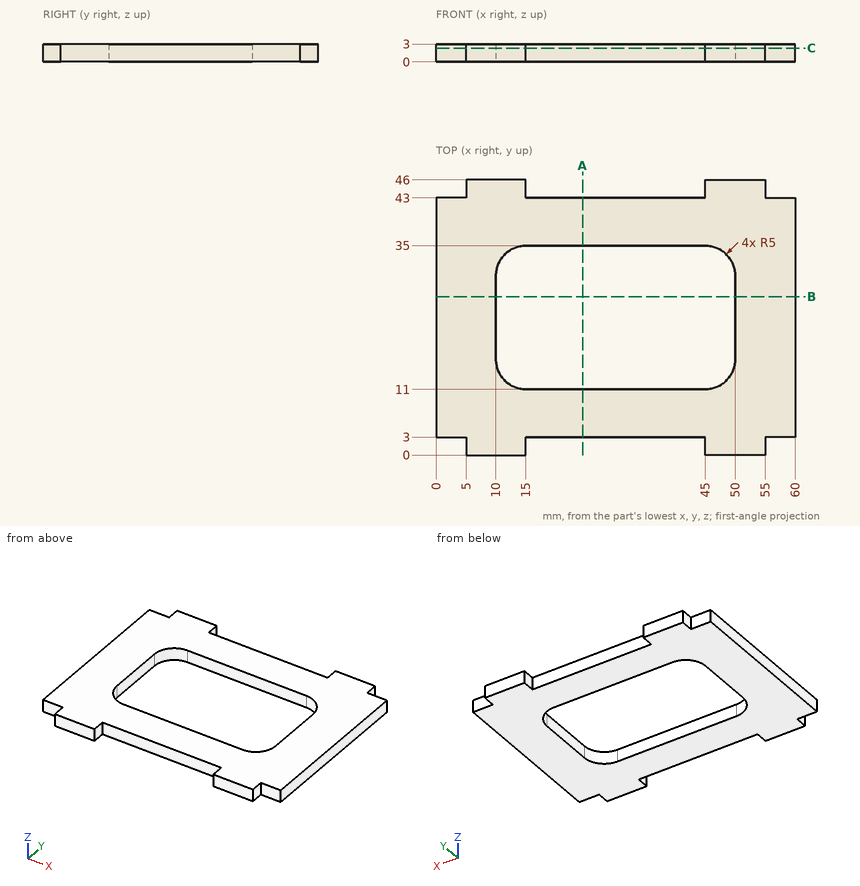
Print and shaded views of the part. All mm, measured from the part's lowest x, y and z. Coordinates: 2 decimals unless noted, no trailing zeros. Order: outer loops, then holes, each group sorted by start corner. A loop starts at its lowest first (then second) coordinate and runs counter-clockwise, first axis right, second up. Notation, with made-up numbers: (46.5, -21) - (64.5, -21) arc R14 cw to (64.5, -10) - close; hole circle Ø2 at (-6, 71.5). An arc over 180 degrees is marked (long way). Return JSON: item names as keys, results as strings. Group by question number.
Item 1: Cut at C-C (z = 2.3). List the corners of the cut face in (x, y).
Item 2: Drill centre lines: probe 1 along X at (y, z) = (23.5, 0.5); probe 2 along Y at (x, z) = (17.5, 0.85); probe 3 along X at (y, z) = (44, 0.9). Where is each one in solid material? Low to high. Write a range as from..to.
Item 3: Cut at B-B (y = 26.5). List the corners of the cut face in (x, z), plus the area to 3 significant figures.
Item 4: Pin check, flat tips, straight feed: pin 1 (1.5 mm diameter, centred on y = 1.5, z = 2, fed in from +X); pin 2 (1.5 mm diameter, centred on x = 37.5, z = 1.5, fed in from -Y). Stop position of each tip, or through.
Item 5: Cut at A-A (x = 24.5). List the corners of the cut face in (y, z).
Check values:
{
 "1": {"outline": "(0, 3) - (5, 3) - (5, 0) - (15, 0) - (15, 3) - (45, 3) - (45, 0) - (55, 0) - (55, 3) - (60, 3) - (60, 43) - (55, 43) - (55, 46) - (45, 46) - (45, 43) - (15, 43) - (15, 46) - (5, 46) - (5, 43) - (0, 43) - close; hole (10, 16) arc R5 ccw to (15, 11) - (45, 11) arc R5 ccw to (50, 16) - (50, 30) arc R5 ccw to (45, 35) - (15, 35) arc R5 ccw to (10, 30) - close"},
 "2": {"probe 1": "x = 0..10, 50..60", "probe 2": "y = 3..11, 35..43", "probe 3": "x = 5..15, 45..55"},
 "3": {"outline": "(0, 0) - (10, 0) - (10, 3) - (0, 3) - close; (50, 0) - (60, 0) - (60, 3) - (50, 3) - close", "area": "60.0 mm2"},
 "4": {"pin 1": "stops at x = 55", "pin 2": "stops at y = 3"},
 "5": {"outline": "(3, 0) - (11, 0) - (11, 3) - (3, 3) - close; (35, 0) - (43, 0) - (43, 3) - (35, 3) - close"}
}
